The model under review builds one solid part; all positions refer to its coordinate system, in mm. A direction names the side the tool comes from. Round coordinates to 2 decimals unless told otherwise and drop trailing zeros. Loops run counter-clockwise (first coordinate to the right, second up) from the corner with the lowest first, then second, coordinate; pieces in that order, holes last. Notation, with made-up numbers: M 3,70.5 L 34,70.5 A33 ccw 34,108.5 Z; hole C 37.5,47 d9. An arc over 180 degrees is marked long. Return JSON: item names as keys, results as strings. Group by question number.
Q1. To check wall thickness, follow line 1 along Y through (x, z) = (32.5, 26.5); line 2 along Z through (x, y) = (-19.5, -70.5); line 3 along X through (y, z) = (73.5, 155.5). State the ranges of each line that lie inside material, in increasing order.
Q2. Consider section C-C (y = -43.5). State the section outline as (x, z) points, and give its area (3 significant figures).
Q3. Consider section B-B (z = 123). State the section outline as (x, y) points, and give its area (3 significant figures).
Q4. Consider section A-A (x = -10.5). State the section outline as (y, z) points.
Q5. For faces 4 (the face through (1, 80, 114)), 5 (the face through (0, -81, 220)), list the 3-axis set-ups (+Z, -Z, +X, -X, +Y, -Y) from which the entire face can be reached by the end or side of a thin tool; tool diameter is ignored.
Q6. Draft analysis for pull direction Z (two halves, no side actions). For faces 1 (the face through (-1, 1, 5)), 2 (the face through (-1, 1, 0)), 3 (the face through (-99.99, -1.42, 108.46)), state which applies: pulls with the +Z half, pulls with the -Z half, needs draft (parallel to the pull), parting line crosses it, or undercut.
Q7. Clearance check with flat-ended pins moving along their axes: pin 1 Ø1 at (y, z) = (-12.5, 116) entering from +X; pin 2 Ø6 at (y, z) = (10, 52) entering from +X; pin 3 Ø1.5 at (x, y) = (1.5, -43) entering from +Z. State where each tip first meets the part, or that it passes through.
Autodesk Inventor part; units mm, degrees
ref_plane "YZ Plane" through (0, 0, 0) normal (1, 0, 0) x (0, 1, 0)
ref_plane "XZ Plane" through (0, 0, 0) normal (0, 1, 0) x (-1, 0, 0)
ref_plane "XY Plane" through (0, 0, 0) normal (0, 0, 1) x (1, 0, 0)
sketch "Sketch1" plane through (0, 0, 0) normal (0, 0, 1) x (1, 0, 0)
  circle A0 centre (0, 0) radius 100
  dimension "d0" = 200
extrude "Extrusion1" add sketch "Sketch1" along normal blind 220
sketch "Sketch3" plane through (0, 0, 220) normal (0, 0, 1) x (1, 0, 0)
  line L0 (0, 0) -> (0, 85) construction
  circle A0 centre (0, 0) radius 100
  arc A1 (52.6783, 85) -> (-52.6783, 85) centre (0, 0) ccw
  line L1 (52.6783, 85) -> (-52.6783, 85)
  dimension "d4" = 85
extrude "Extrusion2" cut sketch "Sketch3" against normal up to surface (220 mm away) contours L1 A0 picked at (-13.4735, 87.1556)
mirror "Mirror1" about plane through (0, 0, 0) normal (0, 1, 0) of "Extrusion2"
shell "Shell1" thickness 5 removed faces 1 at (-13.8939, 25.7023, 220)
properties part number "alternate brain box"
Values:
{
 "1": {"line 1": "y = -85 to -80, 80 to 85", "line 2": "z = 0 to 5", "line 3": "x = -67.81 to -60.19, 60.19 to 67.81"},
 "2": {"outline": "M -90.04,0 L 90.04,0 L 90.04,220 L 84.46,220 L 84.46,5 L -84.46,5 L -84.46,220 L -90.04,220 Z", "area": "3,300 mm2"},
 "3": {"outline": "M -52.68,-85 L 52.68,-85 A100 ccw 52.68,85 L -52.68,85 A100 ccw Z; hole M -51.23,-80 L 51.23,-80 A95 ccw 51.23,80 L -51.23,80 A95 ccw Z", "area": "3,010 mm2"},
 "4": {"outline": "M -85,0 L 85,0 L 85,220 L 80,220 L 80,5 L -80,5 L -80,220 L -85,220 Z"},
 "5": {"face 4": "+Z", "face 5": "+Z, +X, -X, +Y, -Y"},
 "6": {"face 1": "pulls with the +Z half", "face 2": "pulls with the -Z half", "face 3": "needs draft"},
 "7": {"pin 1": "stops at x = 99.28", "pin 2": "stops at x = 99.75", "pin 3": "stops at z = 5"}
}
